Autodesk Inventor part; units mm, degrees
ref_plane "YZ Plane" through (0, 0, 0) normal (1, 0, 0) x (0, 1, 0)
ref_plane "XZ Plane" through (0, 0, 0) normal (0, 1, 0) x (-1, 0, 0)
ref_plane "XY Plane" through (0, 0, 0) normal (0, 0, 1) x (1, 0, 0)
sketch "Sketch3" plane through (0, 0, 0) normal (0, 0, 1) x (1, 0, 0)
  circle A0 centre (14.5794, 0.9769) radius 3.175
  arc A1 (14.5794, -3.4681) -> (19.0244, 0.9769) centre (14.5794, 0.9769) ccw
  line L0 (19.0244, 5.4219) -> (19.0244, 0.9769)
  line L1 (14.5794, 5.4219) -> (19.0244, 5.4219)
  arc A2 (14.5794, 5.4219) -> (10.1344, 0.9769) centre (14.5794, 0.9769) ccw
  line L2 (10.1344, -3.4681) -> (10.1344, 0.9769)
  line L3 (14.5794, -3.4681) -> (10.1344, -3.4681)
  circle A3 centre (14.5794, 0.9769) radius 2.921
  point P0 (0, 0)
  dimension "d3" = 5.842
extrude "Extrusion2" add sketch "Sketch3" against normal blind 6.35 contours A3
sketch "Sketch4" plane through (14.5794, 0.9769, 0) normal (0, 0, 1) x (1, 0, 0)
  circle A0 centre (0, 0) radius 4.191
  circle A1 centre (0, 0) radius 3.175
  arc A2 (0, -4.445) -> (4.445, 0) centre (0, 0) ccw
  line L0 (4.445, 4.445) -> (4.445, 0)
  line L1 (0, 4.445) -> (4.445, 4.445)
  arc A3 (0, 4.445) -> (-4.445, 0) centre (0, 0) ccw
  line L2 (-4.445, -4.445) -> (-4.445, 0)
  line L3 (0, -4.445) -> (-4.445, -4.445)
  circle A4 centre (0, 0) radius 2.921
  point P0 (-14.5794, -0.9769)
  dimension "d6" = 8.382
extrude "Extrusion3" add sketch "Sketch4" against normal blind 3.175 contours A0 | A1 | A4
sketch "Sketch5" plane through (14.5794, 0.9769, 0) normal (0, 0, 1) x (1, 0, 0)
  circle A0 centre (0, 0) radius 4.191
  line L0 (-3.175, -23.495) -> (-3.175, 0)
  line L1 (-3.175, -23.495) -> (3.175, -29.845)
  line L2 (3.175, -29.845) -> (3.175, 0)
  circle A1 centre (0, 0) radius 3.175
  line L3 (3.175, -29.845) -> (-3.175, -23.495)
  point P0 (-14.5794, -0.9769)
  dimension "d9" = 6.35
extrude "Extrusion4" add sketch "Sketch5" against normal blind 3.175 contours L0 A1 L2 A0 | A0 L2 L1 L0 picked at (0.1276, -3.8236)
sketch "Sketch6" plane through (14.5794, 0.9769, -3.175) normal (0, 0, -1) x (-1, 0, 0)
  arc A0 (-4.445, 0) -> (0, -4.445) centre (0, 0) ccw
  line L0 (0, -4.445) -> (23.405, -4.445)
  line L1 (-3.175, -2.7357) -> (-3.175, -29.845)
  line L2 (3.175, -2.7357) -> (3.175, -23.495)
  line L3 (-3.175, -29.845) -> (3.175, -23.495)
  line L4 (3.175, -23.495) -> (3.175, -4.699)
  line L5 (-3.175, -3.4641) -> (-3.175, -29.845)
  arc A1 (0, -4.699) -> (-3.175, -3.4641) centre (0, 0) ccw construction
  line L6 (0, -4.699) -> (3.175, -4.699)
  arc A2 (-3.175, -3.4641) -> (0, -4.699) centre (0, 0) ccw
  point P0 (14.5794, -0.9769)
  dimension "d12" = 9.398
extrude "Extrusion5" add sketch "Sketch6" along normal blind 3.175 contours A2 L6 L2 L3 L1
properties part number "Latch"
Input: part model. Units: mm. Frame: model coordinates. A direction names the side the tool comes from. Give positions to 0.01 mm unless a question says otherwise; leave off trailing zeros. Loops run counter-clockwise (first coordinate to the right, second up) from the corner with the lowest first, then second, coordinate; pieces in that order, holes last. Notation, with made-up numbers: (-19, -16) -> (1, -16) arc R14 ccw to (1, -4) -> close; hole circle Ø8 at (66.25, 14). An arc over 180 degrees is marked (long way). Use a Markdown table: item, result.
Q1. Pull-direction query (Y, two-part tool) for faces 1 (the cylindrical face through (17.366, 1.854, -4.74)), 2 (the cylindrical face through (14.713, 5.166, -1.565)), 3 (the flat face through (15, -15, -6.35)); classes: pulls with the +Y half, pulls with the -Y half, needs draft (parallel to the pull), parting line crosses it, or undercut.
Entries:
| item | result |
|---|---|
| face 1 | undercut |
| face 2 | parting line crosses it |
| face 3 | needs draft |
Q2. Section query A-A, the plane y = 2. Return the cut outline in (x, z) (3 decimals).
Entries:
| item | result |
|---|---|
| outline | (10.515, -3.175) -> (11.843, -3.175) -> (11.843, -6.35) -> (17.315, -6.35) -> (17.315, -3.175) -> (18.644, -3.175) -> (18.644, 0) -> (10.515, 0) -> close |
Q3. Ray query, probe 1 along X at (y, z) = (-13.5, -6); probe 2 along Y at (x, z) = (12.5, -3.5); probe 3 along Y at (x, z) = (12, -3.75). Return the intervals inside material, ascending. Write a range as from..to.
Entries:
| item | result |
|---|---|
| probe 1 | x = 11.4..17.75 |
| probe 2 | y = -23.61..-3.72, -1.07..3.03 |
| probe 3 | y = -23.11..-3.72, -0.39..2.35 |
Q4. Section query D-D, the plane z = -2.5. Return the cut outline in (x, y).
Entries:
| item | result |
|---|---|
| outline | (11.4, -22.52) -> (17.75, -28.87) -> (17.75, -1.76) arc R4.19 ccw (long way) to (11.4, -1.76) -> close |
Q5. Section query C-C, the plane z = -6. Return the cut outline in (x, y), plus the area to 3 significant figures.
Entries:
| item | result |
|---|---|
| outline | (11.4, -22.52) -> (17.75, -28.87) -> (17.75, -2.49) arc R4.7 cw to (14.58, -3.72) -> (11.4, -3.72) -> close; circle Ø5.84 at (14.58, 0.98) |
| area | 168 mm² |
Q6. Section query B-B, the plane x = 12. Return the cut outline in (y, z) (3 decimals), plus the area to 3 significant figures.
Entries:
| item | result |
|---|---|
| outline | (-23.114, -6.35) -> (-3.722, -6.35) -> (-3.722, -3.175) -> (-0.394, -3.175) -> (-0.394, -6.35) -> (2.348, -6.35) -> (2.348, -3.175) -> (4.28, -3.175) -> (4.28, 0) -> (-23.114, 0) -> close |
| area | 157 mm² |
Q7. First-contact query: P1, Ø4, axis at x = 17, y = -23, coming from the +Z side; P2, Ø1.9, axis at y = -11.5, z = -4.5, coming from the -X side; P3, Ø2.5, axis at x = 13, z = -5, coming from the +Y side; P4, Ø1.5, axis at x = 11.5, z = -1.5, coming from the -Y side. Flat tips, straight axial feed; report the tip coordinate or a pass-through.
Entries:
| item | result |
|---|---|
| P1 | stops at z = 0 |
| P2 | stops at x = 11.4 |
| P3 | stops at y = 3.88 |
| P4 | stops at y = -23.36 |
Q8. Access query for faces 4 (the flat face through (17.754, -15, -3)), 5 (the flat face through (14.5, -2.2, -3.175)), 6 (the flat face through (11.404, -12, -3)). Directions: +Z, -Z, +X, -X, +Y, -Y. A direction counts if a zero-diameter tool reaches every point of the face in a straight line with its end or side. Return the directions, or none.
Entries:
| item | result |
|---|---|
| face 4 | +Z, -Z, +X, -Y |
| face 5 | -Z |
| face 6 | +Z, -Z, -X, -Y |
